The model under review builds one solid part; all positions refer to its coordinate system, in mm. Face numbers are marked on the shaded views. Round coordinates to 2 decimals unless told otherwise and drop trailing zeros. Order: outer loops, then holes, each group sorted by start corner. A loop starts at its lowest first (then second) coordinate and runs counter-clockwise, first axis right, second up.
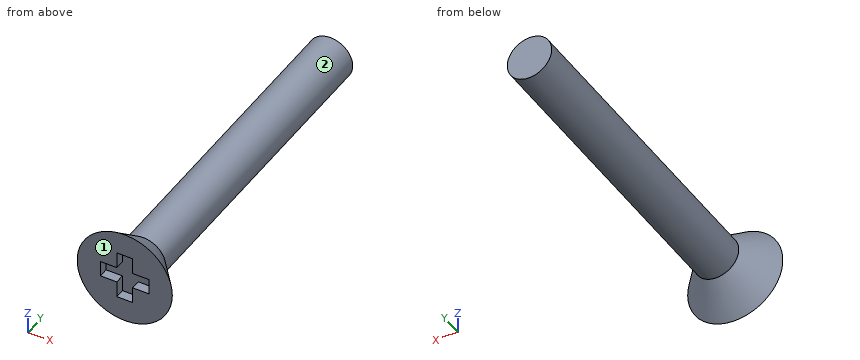
```python
from build123d import *

# Parameters (mm, degrees)
SKETCH_3_R          = 0.7
EXTRUDE_1_DEPTH     = 10
CUT_EXTRUDE_1_DEPTH = 0.3


with BuildPart() as part:
    # 草图2 → 旋转1 (revolve)
    with BuildSketch(Plane.XY):
        Polygon((0, 0), (1.5, 0), (0.7, 1), (0, 1), align=None)
    revolve(axis=Axis((0, 0, 0), (0, 1, 0)))

    # 草图3 → 凸台-拉伸1 (add)
    with BuildSketch(Plane(origin=(0, 1, 0), x_dir=(1, 0, 0), z_dir=(0, 1, 0))):
        Circle(SKETCH_3_R)
    extrude(amount=EXTRUDE_1_DEPTH)

    # 草图4 → 切除-拉伸1 (cut)
    with BuildSketch(Plane.XZ):
        Polygon((0.25, -0.25), (0.25, -0.765105953), (0, -0.765105953), (-0.25, -0.765105953), (-0.25, -0.25), (-0.765105953, -0.25), (-0.765105953, 0), (-0.765105953, 0.25), (-0.25, 0.25), (-0.25, 0.765105953), (0, 0.765105953), (0.25, 0.765105953), (0.25, 0.25), (0.765105953, 0.25), (0.765105953, 0), (0.765105953, -0.25), align=None)
    extrude(amount=-CUT_EXTRUDE_1_DEPTH, mode=Mode.SUBTRACT)


solid = part.part
```
(1) Consider section A-A (x = 0). Write out the cut boundary in (y, z), and give its area (3 significant figures).
Data:
outline: (0, -1.5) - (1, -0.7) - (11, -0.7) - (11, 0.7) - (1, 0.7) - (0, 1.5) - (0, 0.77) - (0.3, 0.77) - (0.3, -0.77) - (0, -0.77) - close
area: 15.7 mm2
(2) Consider section B-B (z = 0). Write out the cut boundary in (x, y).
Data:
outline: (-1.5, 0) - (-0.77, 0) - (-0.77, 0.3) - (0.77, 0.3) - (0.77, 0) - (1.5, 0) - (0.7, 1) - (0.7, 11) - (-0.7, 11) - (-0.7, 1) - close
(3) Consider section C-C (y = 4). Write out the cut boundary in (x, z).
Data:
outline: circle Ø1.4 at (0, 0)
(4) Draft analysis for pull direction Z (two halves, no side actions). For the marked faces 1 and 2, state which applies: pulls with the +Z half, pulls with the -Z half, needs draft (parallel to the pull), parting line crosses it, or undercut.
Data:
face 1: needs draft
face 2: parting line crosses it
(5) To check wall thickness, follow probe 1 along Y at (x, z) = (0, -0.5); probe 2 along X at (y, z) = (7.75, 0.05); probe 3 along X at (y, z) = (5.25, -0.6). State the ranges of each line that lie inside material, in increasing order.
Data:
probe 1: y = 0.3 to 11
probe 2: x = -0.7 to 0.7
probe 3: x = -0.36 to 0.36
(6) Insertion check: pin 1 (1.5 mm diameter, centred on y = 4, z = 0.5, fed in from -X). The pin has a flat end and moves straight along its axis. Give the tip position at first contact, or say it passes through.
Data:
pin 1: stops at x = -0.7
